Here's how the part is built. I have some questions about the finished solid (model axes, mm). Face numbers are marked on the shaded views. A direction names the side the tool comes from. Coordinates: 2 decimals unless noted, no trailing zeros. Loops run counter-clockwise (first coordinate to the right, second up) from the corner with the lowest first, then second, coordinate; pieces in that order, holes last. Notation, with made-up numbers: M 46.25,-10 L 84.25,-10 A26 ccw 84.25,16 Z; hole C -15.75,33 d7. An arc over 180 degrees is marked long. Use CSV: the item, a comma, the result in double quotes. Start each with the question number.
Q1. If we section it at B-B (x = 14): Please give me the cut outline in (y, z).
Q2. Please list where these lines run through material, in increasing order: probe 1 along Y at (x, z) = (35, 2); probe 2 along Y at (x, z) = (60, 19.5); probe 3 along Z at (x, y) = (6.5, 6). Write a range as [from, to].
Q3. If we mould it in two halves opening along Y, with no side actions, what happens to the marked faces 5, 6 and 7? For each: +Y half, -Y half, draft (parallel to the pull), parting line (faces both ways), or undercut.
Q4. For pin 1 Ø14.5 at (x, y) = (35, 0) entering from -Z; pin 2 Ø2 at (y, z) = (-14.5, 12) entering from +X; pin 3 Ø15 at (x, z) = (46, 19) entering from -Y, each with a flat end and sliding along its axis, tell me the tip position at first contact or that it passes through.
Q5. If we section it at D-D (x = 60): Please give me the cut outline in (y, z), and give its area (3 significant figures).
Q6. If we section it at C-C (z = 4.25): Please give me the cut outline in (x, y), and give its area (3 significant figures).
Q7. Which directions (+Z, -Z, +X, -X, +Y, -Y) give clear straight access to the entire face, cutting with the end or side of a thin tool? Please do the marked faces 1, 2, 3 and 4.
Q8. If we section it at A-A (y = 0): State how many separate pieces and enclosed holes the cut face has, and give its area (3 significant figures).
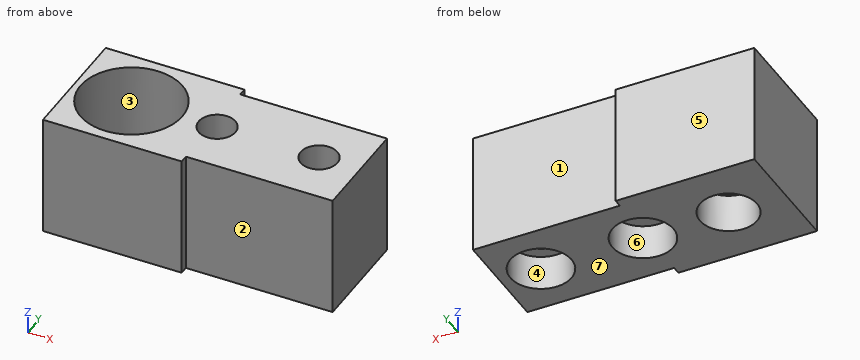
from build123d import *

# Parameters (mm, degrees)
AUFSATZ_LINEAR_AUSTRAGEN1_DEPTH                      = 30
SKIZZE6_R                                            = 12.5
SCHNITT_LINEAR_AUSTRAGEN1_DEPTH                      = 20
M16_GEWINDEBOHRUNG1_D                                = 14
M16_GEWINDEBOHRUNG1_DEPTH                            = 42
M16_GEWINDEBOHRUNG1_TIP                              = 4.206024333
STIRNSENKUNG_F_R_M8_ZYLINDERSCHRAUBE_MIT_D           = 9
STIRNSENKUNG_F_R_M8_ZYLINDERSCHRAUBE_MIT_CBORE_D     = 15
STIRNSENKUNG_F_R_M8_ZYLINDERSCHRAUBE_MIT_CBORE_DEPTH = 8.6
FASE1_SIZE                                           = 0.5


with BuildPart() as part:
    # Skizze1 → Aufsatz-Linear austragen1 (new body)
    with BuildSketch(Plane.XY):
        Polygon((34, 15), (34, 13), (70, 13), (70, -13), (34, -13), (34, -15), (0, -15), (0, 15), align=None)
    extrude(amount=AUFSATZ_LINEAR_AUSTRAGEN1_DEPTH)

    # Skizze6 → Schnitt-Linear austragen1 (cut)
    with BuildSketch(Plane.XY.offset(30)):
        with Locations((14, 0)):
            Circle(SKIZZE6_R)
    extrude(amount=-SCHNITT_LINEAR_AUSTRAGEN1_DEPTH, mode=Mode.SUBTRACT)

    # M16 Gewindebohrung1
    with Locations(Plane(origin=(0, 0, 0), x_dir=(-1, 0, 0), z_dir=(0, 0, -1))):
        with Locations((-14, 0)):
            Hole(M16_GEWINDEBOHRUNG1_D / 2, depth=M16_GEWINDEBOHRUNG1_DEPTH)
            with Locations((0, 0, -(M16_GEWINDEBOHRUNG1_DEPTH + M16_GEWINDEBOHRUNG1_TIP / 2))):  # 118° drill point
                Cone(0, M16_GEWINDEBOHRUNG1_D / 2, M16_GEWINDEBOHRUNG1_TIP, mode=Mode.SUBTRACT)

    # Stirnsenkung für M8 Zylinderschraube mit Innensechskant1 (through all)
    with Locations(Plane(origin=(0, 0, 0), x_dir=(-1, 0, 0), z_dir=(0, 0, -1))):
        with Locations((-60, 0), (-35, 0)):
            CounterBoreHole(STIRNSENKUNG_F_R_M8_ZYLINDERSCHRAUBE_MIT_D / 2, STIRNSENKUNG_F_R_M8_ZYLINDERSCHRAUBE_MIT_CBORE_D / 2, STIRNSENKUNG_F_R_M8_ZYLINDERSCHRAUBE_MIT_CBORE_DEPTH)

    # Fase1
    fase1_edges = [part.edges().sort_by_distance(p)[0] for p in [
        (7, 0, 10),
    ]]
    chamfer(fase1_edges, length=FASE1_SIZE)


solid = part.part
Results below:
1,outline,"M -15,0 L -7,0 L -7,9.5 L -7.5,10 L -12.5,10 L -12.5,30 L -15,30 Z; M 7,0 L 15,0 L 15,30 L 12.5,30 L 12.5,10 L 7.5,10 L 7,9.5 Z"
2,probe 1,"[-13, -7.5], [7.5, 13]"
2,probe 2,"[-13, -4.5], [4.5, 13]"
2,probe 3,"[0, 10]"
3,face 5,"+Y half"
3,face 6,"undercut"
3,face 7,"draft"
4,pin 1,"z = 8.6"
4,pin 2,"x = 34"
4,pin 3,"y = -13"
5,outline,"M -13,0 L -7.5,0 L -7.5,8.6 L -4.5,8.6 L -4.5,30 L -13,30 Z; M 4.5,8.6 L 7.5,8.6 L 7.5,0 L 13,0 L 13,30 L 4.5,30 Z"
5,area,"458 mm^2"
6,outline,"M 0,-15 L 34,-15 L 34,-13 L 70,-13 L 70,13 L 34,13 L 34,15 L 0,15 Z; hole C 14,0 d14; hole C 35,0 d15; hole C 60,0 d15"
6,area,"1,450 mm^2"
7,face 1,"+Z, -Z, +X, +Y"
7,face 2,"+Z, -Z, +X, -Y"
7,face 3,"+Z"
7,face 4,"-Z"
8,separate pieces,"4"
8,enclosed holes,"0"
8,area,"817 mm^2"
